Read the model definition and answer for the solid it produces. Units are mm, in the model's axes. Round coordinates to 2 decimals unless told otherwise and drop trailing zeros. Order: outer loops, then holes, each group sorted by start corner. A loop starts at its lowest first (then second) coordinate and runs counter-clockwise, first axis right, second up. Notation, with made-up numbers: (80.5, 32) -> (116.5, 32) arc R23 ccw to (116.5, 47) -> close; hole circle Ø2 at (45, 13.25). An arc over 180 degrees is marked (long way). One line per item, written item: value. Start each with the question number.
1. Section A-A (z = 0.7) is taken. State how many separate pieces and enclosed holes the cut face has, then the cut area to 3 significant figures.
2. Flat-ended cylindrical pins translate along their axes: pin 1 Ø5 at (x, y) = (-95.02, 0) entering from -Z; pin 2 Ø5 at (x, y) = (88, 133) entering from -Z; pin 3 Ø0.5 at (x, z) = (-140.5, 0.5) entering from -Y; pin 4 Ø0.5 at (y, z) = (-11, 0.5) entering from +X. Find the tip coordinate at first contact, or state that the pin passes through.
3. Section B-B (x = -116) is taken. Give the vertices of the cut face in (y, z), then the cut area to 3 significant figures.
4. Consider line 1 (Y direction, x = -103, z = 0.75); line 2 (X direction, y = -8, z = 0.05). Determine where each line is inside the solid, lowest interval first.
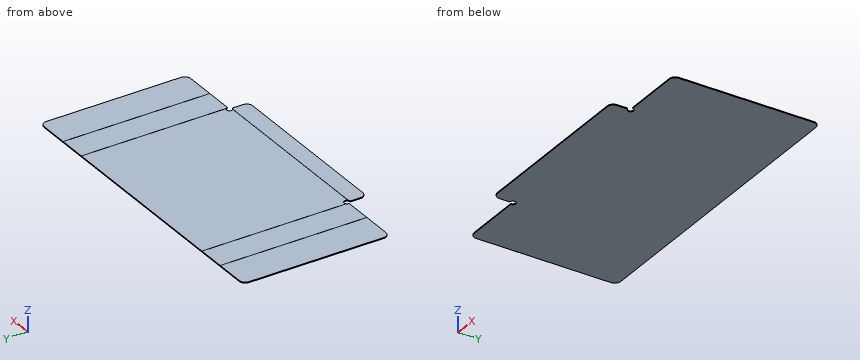
from build123d import *

# Parameters (mm, degrees)
F0_W     = 190.0428
F0_H     = 2.1717
F0_W_2   = 0.127
F0_H_2   = 152.4
F0_H_3   = 0.127
F1_DEPTH = 1.016
F2_W     = 0.127
F2_H     = 152.4
F2_W_2   = 190.0428
F2_H_2   = 0.127
F3_DEPTH = 0.508
F5_D     = 6.35


with BuildPart() as f1:
    # F0 (on Top) → F1 (new body)
    with BuildSketch(Plane.XY):
        Polygon((-97.1931, 0), (-95.0214, 0), (95.0214, 0), (97.1931, 0), (97.1931, 152.4), (95.0214, 152.4), (-95.0214, 152.4), (-97.1931, 152.4), align=None)
        with Locations((0, -1.08585)):
            Rectangle(F0_W, F0_H)
        with Locations((-97.2566, 76.2)):
            Rectangle(F0_W_2, F0_H_2)
        with Locations((0, -2.2352)):
            Rectangle(F0_W, F0_H_3)
        with Locations((97.2566, 76.2)):
            Rectangle(F0_W_2, F0_H_2)
        Polygon((-99.4918, 0), (-97.3201, 0), (-97.3201, 152.4), (-99.4918, 152.4), (-124.4346, 152.4), (-126.6063, 152.4), (-126.6063, 0), (-124.4346, 0), align=None)
        with Locations((0, -3.38455)):
            Rectangle(F0_W, F0_H)
        Polygon((97.3201, 152.4), (97.3201, 0), (99.4918, 0), (124.4346, 0), (126.6063, 0), (126.6063, 152.4), (124.4346, 152.4), (99.4918, 152.4), align=None)
        with BuildLine():
            Line((95.0214, -4.4704), (-95.0214, -4.4704))
            Line((-95.0214, -4.4704), (-95.0214, -13.7668))
            ThreePointArc((-95.0214, -13.7668), (-93.161528, -18.256928), (-88.6714, -20.1168))
            Line((-88.6714, -20.1168), (88.6714, -20.1168))
            ThreePointArc((88.6714, -20.1168), (93.161528, -18.256928), (95.0214, -13.7668))
            Line((95.0214, -13.7668), (95.0214, -4.4704))
        make_face()
        with Locations((-126.6698, 76.2)):
            Rectangle(F0_W_2, F0_H_2)
        with Locations((126.6698, 76.2)):
            Rectangle(F0_W_2, F0_H_2)
        with BuildLine():
            Line((-128.905, 0), (-126.7333, 0))
            Line((-126.7333, 0), (-126.7333, 152.4))
            Line((-126.7333, 152.4), (-128.905, 152.4))
            Line((-128.905, 152.4), (-157.2514, 152.4))
            ThreePointArc((-157.2514, 152.4), (-161.741528, 150.540128), (-163.6014, 146.05))
            Line((-163.6014, 146.05), (-163.6014, 6.35))
            ThreePointArc((-163.6014, 6.35), (-161.741528, 1.859872), (-157.2514, 0))
            Line((-157.2514, 0), (-128.905, 0))
        make_face()
        with BuildLine():
            Line((126.7333, 152.4), (126.7333, 0))
            Line((126.7333, 0), (128.905, 0))
            Line((128.905, 0), (157.2514, 0))
            ThreePointArc((157.2514, 0), (161.741528, 1.859872), (163.6014, 6.35))
            Line((163.6014, 6.35), (163.6014, 146.05))
            ThreePointArc((163.6014, 146.05), (161.741528, 150.540128), (157.2514, 152.4))
            Line((157.2514, 152.4), (128.905, 152.4))
            Line((128.905, 152.4), (126.7333, 152.4))
        make_face()
    extrude(amount=F1_DEPTH)

    # F2 (on face) → F3 (cut)
    with BuildSketch(Plane.XY.offset(1.016)):
        with Locations((-126.6698, 76.2)):
            Rectangle(F2_W, F2_H)
        with Locations((-97.2566, 76.2)):
            Rectangle(F2_W, F2_H)
        with Locations((97.2566, 76.2)):
            Rectangle(F2_W, F2_H)
        with Locations((126.6698, 76.2)):
            Rectangle(F2_W, F2_H)
        with Locations((0, -2.2352)):
            Rectangle(F2_W_2, F2_H_2)
    extrude(amount=-F3_DEPTH, mode=Mode.SUBTRACT)

    # F5 (through all)
    with Locations(Plane.XY.offset(1.016)):
        with Locations((95.0214, 0), (-95.0214, 0)):
            Hole(F5_D / 2)


solid = f1.part
Answer:
1. separate pieces: 6
1. enclosed holes: 0
1. area: 53,500 mm^2
2. pin 1: through
2. pin 2: z = 0
2. pin 3: y = 0
2. pin 4: x = 95.02
3. outline: (0, 0) -> (152.4, 0) -> (152.4, 1.02) -> (0, 1.02) -> close
3. area: 155 mm^2
4. line 1: 0 to 152.4
4. line 2: -95.02 to 95.02
